The model under review builds one solid part; all positions refer to its coordinate system, in mm. Face numbers are marked on the shaded views. A direction names the side the tool comes from. Coordinates: 2 decimals unless noted, no trailing zeros. Write each loop counter-clockwise with the first axis right and the second up, starting at its lowest first coordinate (ties: lowest second). Pieces come first, ordered by that corner, then holes. Notation, with made-up numbers: (-18.5, 87) - (10.5, 87) arc R29 ccw to (10.5, 107) - close; hole circle Ø5 at (20, 58.25). An arc over 180 degrees is marked (long way). Return JSON: item names as keys, results as strings. Group by question number.
(1) We need section B-B on z = 15.57. State the section outline as (x, y) points (3 decimals), then the cut area to 3 significant figures.
(2) We need section C-C on z = 29. State the section outline as (x, y) points.
(3) We need section D-D on y = 12.75. State the section outline as (x, z) points, then the cut area to 3 significant figures.
(4) Tool access review of the marked faces 1, 2 and 3: name each direction out of +Z, -Z, +X, -X, +Y, -Y from which nothing blocks a thin tool from reaching the whole face with its end or side.
(5) To check wall thickness, follow L1, parallel to Z at x = 62, y = 24; L2, parallel to X at y = 4.5, z = 4.9 (3 decimals); L3, parallel to Y at x = 3.5, z = 15.57 (3 decimals). State the ranges of each line that lie inside material, in increasing order. Write a range as from..to.
(6) We need section A-A on x = 118.5. State the section outline as (y, z) points (3 decimals).
(7) For pin 1 Ø6.5 at (y, z) = (20.72, 64.43) entering from +X; pin 2 Ø11 at (y, z) = (19.5, 13.5) entering from +X; pin 3 Ø8.5 at (x, z) = (118.5, 75.1) entering from +Y, all flat-tipped, find the tip position at first contact; note any pin that passes through.
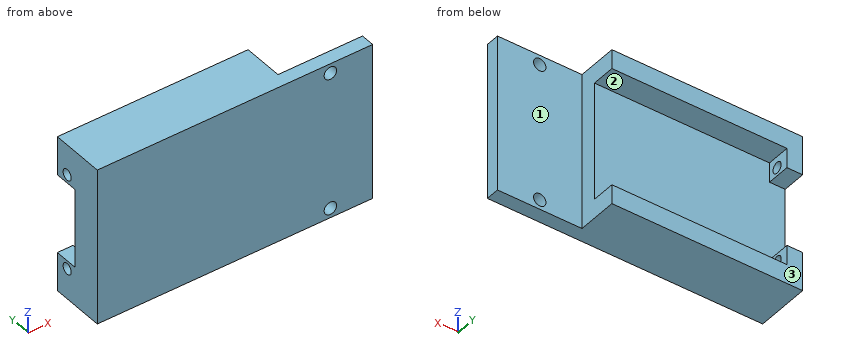
```python
from build123d import *

# Parameters (mm, degrees)
BOSS_EXTRUDE1_DEPTH = 80
BOSS_EXTRUDE2_DEPTH = 12
SKETCH3_R           = 2.795
CUT_EXTRUDE1_DEPTH  = 60
SKETCH4_R           = 3.175
CUT_EXTRUDE2_DEPTH  = 10


with BuildPart() as part:
    # Sketch1 → Boss-Extrude1 (new body)
    with BuildSketch(Plane.XY):
        Polygon((140, 0), (0, 0), (0, 15.49), (97, 15.49), (97, 6.96), (140, 6.96), align=None)
    extrude(amount=BOSS_EXTRUDE1_DEPTH)

    # Sketch2 → Boss-Extrude2 (add)
    with BuildSketch(Plane(origin=(0, 15.49, 0), x_dir=(1, 0, 0), z_dir=(0, 1, 0))):
        Polygon((97, 0), (0, 0), (0, -9.8), (0, -19.8), (8, -19.8), (8, -9.8), (97, -9.8), align=None)
        Polygon((8, -60.2), (0, -60.2), (0, -70.2), (0, -80), (97, -80), (97, -70.2), (8, -70.2), align=None)
    extrude(amount=BOSS_EXTRUDE2_DEPTH)

    # Sketch3 → Cut-Extrude1 (cut)
    with BuildSketch(Plane.ZY):
        with Locations((15.57, 20.72)):
            Circle(SKETCH3_R)
        with Locations((64.43, 20.72)):
            Circle(SKETCH3_R)
    extrude(amount=-CUT_EXTRUDE1_DEPTH, mode=Mode.SUBTRACT)

    # Sketch4 → Cut-Extrude2 (cut)
    with BuildSketch(Plane(origin=(0, 6.96, 0), x_dir=(1, 0, 0), z_dir=(0, 1, 0))):
        with Locations(Location((118.5, -4.9, 0), (0, 0, 270))):
            Circle(SKETCH4_R)
        with Locations(Location((118.5, -75.1, 0), (0, 0, 270))):
            Circle(SKETCH4_R)
    extrude(amount=-CUT_EXTRUDE2_DEPTH, mode=Mode.SUBTRACT)


solid = part.part
```
Ans:
{
 "1": {"outline": "(0, 0) - (140, 0) - (140, 6.96) - (97, 6.96) - (97, 15.49) - (8, 15.49) - (8, 17.925) - (0, 17.925) - close; (0, 23.515) - (8, 23.515) - (8, 27.49) - (0, 27.49) - close", "area": "1,850 mm²"},
 "2": {"outline": "(0, 0) - (140, 0) - (140, 6.96) - (97, 6.96) - (97, 15.49) - (0, 15.49) - close"},
 "3": {"outline": "(0, 0) - (97, 0) - (97, 80) - (0, 80) - close", "area": "7,760 mm²"},
 "4": {"face 1": "+Z, -Z, +X, +Y", "face 2": "+X, +Y", "face 3": "+Z, -Z, +X, -X, +Y"},
 "5": {"L1": "0..9.8, 70.2..80", "L2": "0..115.325, 121.675..140", "L3": "0..17.925, 23.515..27.49"},
 "6": {"outline": "(0, 0) - (6.96, 0) - (6.96, 1.725) - (0, 1.725) - close; (0, 8.075) - (6.96, 8.075) - (6.96, 71.925) - (0, 71.925) - close; (0, 78.275) - (6.96, 78.275) - (6.96, 80) - (0, 80) - close"},
 "7": {"pin 1": "x = 8", "pin 2": "x = 97", "pin 3": "y = 6.96"}
}
